from build123d import *

# Parameters (mm, degrees)
ESQUISSE1_R             = 2.046773471
BOSS_EXTRU_1_DEPTH      = 3.3
BOSS_EXTRU_2_DEPTH      = 1.3
BOSS_EXTRU_2_DEPTH_BACK = 4.6
ESQUISSE2_R             = 2.046773471
CHANFREIN1_SIZE         = 5
CHANFREIN1_SIZE_2       = 1.3
CHANFREIN3_SIZE         = 5
CHANFREIN3_SIZE_2       = 1.3
CHANFREIN2_SIZE         = 1
ESQUISSE3_R             = 5.5
ESQUISSE3_R_2           = 2.75
BOSS_EXTRU_3_DEPTH      = 1.8
CHANFREIN4_SIZE         = 1.5
ESQUISSE4_R             = 3.5
ENL_V_MAT_EXTRU_1_DEPTH = 3.5
CHANFREIN5_SIZE         = 1.3
ESQUISSE5_R             = 0.75
ENL_V_MAT_EXTRU_2_DEPTH = 3.5


with BuildPart() as part:
    # Esquisse1 → Boss.-Extru.1 (new body)
    with BuildSketch(Plane.XY):
        with BuildLine():
            Line((0.875, 6.945097192), (24.5, 3.968626967))
            ThreePointArc((24.5, 3.968626967), (28, 0), (24.5, -3.968626967))
            Line((24.5, -3.968626967), (0.875, -6.945097192))
            ThreePointArc((0.875, -6.945097192), (-7, 0), (0.875, 6.945097192))
        make_face()
        Circle(ESQUISSE1_R, mode=Mode.SUBTRACT)
    extrude(amount=BOSS_EXTRU_1_DEPTH)

    # Esquisse2 → Boss.-Extru.2 (add, two sides: drawn at the far end of the back side and taken through both)
    with BuildSketch(Plane.XY.offset(3.3).offset(-BOSS_EXTRU_2_DEPTH_BACK)):
        with BuildLine():
            Line((0.875, 6.945097192), (6.5, 6.236413805))
            Line((6.5, 6.236413805), (6.5, -6.236413805))
            Line((6.5, -6.236413805), (0.875, -6.945097192))
            ThreePointArc((0.875, -6.945097192), (-7, 0), (0.875, 6.945097192))
        make_face()
        Circle(ESQUISSE2_R, mode=Mode.SUBTRACT)
    extrude(amount=BOSS_EXTRU_2_DEPTH + BOSS_EXTRU_2_DEPTH_BACK)

    # Chanfrein1
    # the kernel refuses this chamfer: 5, 1.3 mm, written as the material it adds along each edge
    with BuildSketch(Plane(origin=(6.5, 19.22093464, 3.3), x_dir=(0.9999530531472482, 0, -0.009689762716214913), z_dir=(0, -1, 0))) as chanfrein1_piece_1_section:
        Polygon((CHANFREIN1_SIZE * 0.999953053147, CHANFREIN1_SIZE * 0.00968976271621), (-CHANFREIN1_SIZE_2 * 0.00968976271621, CHANFREIN1_SIZE_2 * 0.999953053147), (0, 0), align=None)
    chanfrein1_piece_1 = extrude(amount=38.441869281, mode=Mode.PRIVATE)
    chanfrein1_piece_1 = split(chanfrein1_piece_1, bisect_by=Plane(origin=(8.958471047, 5.926675567, 3.684204829), z_dir=(-0.12500000000000006, -0.9921567416492215, 0)), keep=Keep.TOP, mode=Mode.PRIVATE)
    chanfrein1_piece_1 = split(chanfrein1_piece_1, bisect_by=Plane(origin=(8.958471047, -5.926675567, 3.684204829), z_dir=(-0.1249999999999999, 0.9921567416492215, 0)), keep=Keep.TOP, mode=Mode.PRIVATE)
    chanfrein1_piece_1 = split(chanfrein1_piece_1, bisect_by=Plane(origin=(8.211780112, 0, 4.6), z_dir=(0, 0, -1)), keep=Keep.TOP, mode=Mode.PRIVATE)
    add(chanfrein1_piece_1)

    # Chanfrein3
    # the kernel refuses this chamfer: 5, 1.3 mm, written as the material it adds along each edge
    with BuildSketch(Plane(origin=(6.5, 19.22093464, 0), x_dir=(0.9999530531472482, 0, 0.009689762716214958), z_dir=(0, -1, 0))) as chanfrein3_piece_1_section:
        Polygon((CHANFREIN3_SIZE * 0.999953053147, -CHANFREIN3_SIZE * 0.00968976271621), (-CHANFREIN3_SIZE_2 * 0.00968976271621, -CHANFREIN3_SIZE_2 * 0.999953053147), (0, 0), align=None)
    chanfrein3_piece_1 = extrude(amount=38.441869281, mode=Mode.PRIVATE)
    chanfrein3_piece_1 = split(chanfrein3_piece_1, bisect_by=Plane(origin=(8.958471047, 5.926675567, -0.384204829), z_dir=(-0.1250000000000275, -0.9921567416492181, 0)), keep=Keep.TOP, mode=Mode.PRIVATE)
    chanfrein3_piece_1 = split(chanfrein3_piece_1, bisect_by=Plane(origin=(8.958471047, -5.926675567, -0.384204829), z_dir=(-0.1250000000000275, 0.9921567416492181, 0)), keep=Keep.TOP, mode=Mode.PRIVATE)
    chanfrein3_piece_1 = split(chanfrein3_piece_1, bisect_by=Plane(origin=(8.211780112, 0, -1.3), z_dir=(0, 0, 1)), keep=Keep.TOP, mode=Mode.PRIVATE)
    add(chanfrein3_piece_1)

    # Chanfrein2
    chanfrein2_edges = [part.edges().sort_by_distance(p)[0] for p in [
        (-7, 0, -1.3),
        (3.6875, 6.590755498, -1.3),
        (3.6875, -6.590755498, -1.3),
        (-7, 0, 4.6),
        (3.6875, -6.590755498, 4.6),
        (3.6875, 6.590755498, 4.6),
    ]]
    chamfer(chanfrein2_edges, length=CHANFREIN2_SIZE)

    # Esquisse3 → Boss.-Extru.3 (add)
    with BuildSketch(Plane(origin=(0, 0, -1.3), x_dir=(-1, 0, 0), z_dir=(0, 0, -1))):
        with Locations(Location((0, 0, 0), (0, 0, 180))):
            Circle(ESQUISSE3_R)
        Circle(ESQUISSE3_R_2, mode=Mode.SUBTRACT)
    extrude(amount=BOSS_EXTRU_3_DEPTH)

    # Chanfrein4
    chanfrein4_edges = [part.edges().sort_by_distance(p)[0] for p in [
        (-5.5, 0, -3.1),
    ]]
    chamfer(chanfrein4_edges, length=CHANFREIN4_SIZE)

    # Esquisse4 → Enlèv. mat.-Extru.1 (cut)
    with BuildSketch(Plane.XY.offset(4.6)):
        Circle(ESQUISSE4_R)
    extrude(amount=-ENL_V_MAT_EXTRU_1_DEPTH, mode=Mode.SUBTRACT)

    # Chanfrein5
    chanfrein5_edges = [part.edges().sort_by_distance(p)[0] for p in [
        (-3.5, 0, 4.6),
    ]]
    chamfer(chanfrein5_edges, length=CHANFREIN5_SIZE)

    # Esquisse5 → Enlèv. mat.-Extru.2 (cut)
    with BuildSketch(Plane.XY.offset(3.3)):
        with Locations((24, 0)):
            Circle(ESQUISSE5_R)
        with Locations((20, 0)):
            Circle(ESQUISSE5_R)
    extrude(amount=-ENL_V_MAT_EXTRU_2_DEPTH, mode=Mode.SUBTRACT)


solid = part.part
Can you work these out from the model? Positions are in its coordinate system, mm. A direction names the side the tool comes from. Coordinates: 2 decimals unless noted, no trailing zeros. Loops run counter-clockwise (first coordinate to the right, second up) from the corner with the lowest first, then second, coordinate; pieces in that order, holes last. Notation, with made-up numbers: M 25.5,34.25 L 60.5,34.25 A24 cw 60.5,71.25 Z; hole C 65.5,-34.75 d9. An arc over 180 degrees is marked long. Return JSON: item names as keys, results as strings. Group by question number.
Item 1: If I drill on L1, parallel to Y at x = 0, z = 2.5; L2, parallel to Y at x = 0, z = -1.85; L3, parallel to Z at x = 16.5, y = -3.5, over which ranges is the centre line in solid material (lowest first)? Write a range as from..to.
Item 2: Thinking about a two-plate mould opening in X: for faces 5 (the flat face through (3.66, -6.08, 4.11)), 6 (the cylindrical face through (3.233, -1.341, 2.215)), 7 (the flat face through (-1, 3, -3.1)), which applies, released by +X, released by -X, zero draft, split by the parting line, or undercut?
Item 3: Imagine slicing it at C-C (y = 0). Give the number of separate pieces and of enclosed holes in the cut face, and give its area (3 significant figures).
Item 4: I'm going to push flat-ended pins straight in: pin 1 Ø3.5 at (x, y) = (0, 1.5) entering from +Z; pin 2 Ø2 at (x, y) = (20, 0) entering from -Z; pin 3 Ø1 at (y, z) = (-5.5, -1) entering from -X. Where does each tip first touch, or does it pass through?
Item 5: Imagine slicing it at B-B (z = 1.75). Please give me the cut outline in (x, y) (3 decimals), and give its area (3 significant figures).
Item 6: On a 3-axis mill with a long thin cutter (end or side, diameter ignored), from which of +Z, -Z, +X, -X, +Y, -Y can I reach the whole of each face in a straight line? I mean faces 1 (the flat face through (9.035, 0.081, -0.641)), 2 (the flat face through (2, -1, -1.3)), 3 (the flat face through (18, 0, 3.3)), 4 (the flat face through (2, -2, 1.1)). Say none if no direction works.
Item 7: Imagine slicing it at A-A (x = 0). Please give me the cut outline in (y, z).
Item 8: Imagine slicing it at D-D (x = 24). Please give me the cut outline in (y, z).
Verdict:
{
 "1": {"L1": "y = -7..-3.5, 3.5..7", "L2": "y = -5.25..-2.75, 2.75..5.25", "L3": "z = 0..3.3"},
 "2": {"face 5": "released by +X", "face 6": "undercut", "face 7": "zero draft"},
 "3": {"separate pieces": "4", "enclosed holes": "0", "area": "118 mm^2"},
 "4": {"pin 1": "stops at z = 1.1", "pin 2": "stops at z = 0", "pin 3": "stops at x = -4.23"},
 "5": {"outline": "M 0.875,-6.945 L 24.5,-3.969 A4 ccw 24.5,3.969 L 0.875,6.945 A7 ccw long Z; hole C 0,0 d7; hole C 20,0 d1.5; hole C 24,0 d1.5", "area": "326 mm^2"},
 "6": {"face 1": "-Z, +X, +Y, -Y", "face 2": "-Z", "face 3": "+Z, +X, +Y, -Y", "face 4": "+Z"},
 "7": {"outline": "M -7,-0.3 L -6,-1.3 L -5.5,-1.3 L -5.5,-1.6 L -4,-3.1 L -2.75,-3.1 L -2.75,-1.3 L -2.05,-1.3 L -2.05,1.1 L -3.5,1.1 L -3.5,3.3 L -4.8,4.6 L -6,4.6 L -7,3.6 Z; M 2.05,-1.3 L 2.75,-1.3 L 2.75,-3.1 L 4,-3.1 L 5.5,-1.6 L 5.5,-1.3 L 6,-1.3 L 7,-0.3 L 7,3.6 L 6,4.6 L 4.8,4.6 L 3.5,3.3 L 3.5,1.1 L 2.05,1.1 Z"},
 "8": {"outline": "M -4.03,0 L -0.75,0 L -0.75,3.3 L -4.03,3.3 Z; M 0.75,0 L 4.03,0 L 4.03,3.3 L 0.75,3.3 Z"}
}
